Part print with two shaded views. Sizes in mm from the minimum x, y, z corner. A direction names the side the tool comes from. Give positions to 0.01 mm unless a question says otherwise; leave off trailing zeros. Order: outer loops, then holes, each group sorted by start corner. A loop starts at its lowest first (then second) coordinate and runs counter-clockwise, first axis right, second up. Notation, with made-up numbers: M -27,14 L 17,14 A13 ccw 17,20 Z; hole C 36.25,74.25 d8. An arc over 180 degrees is marked long. Answer as CSV lines item,"result".
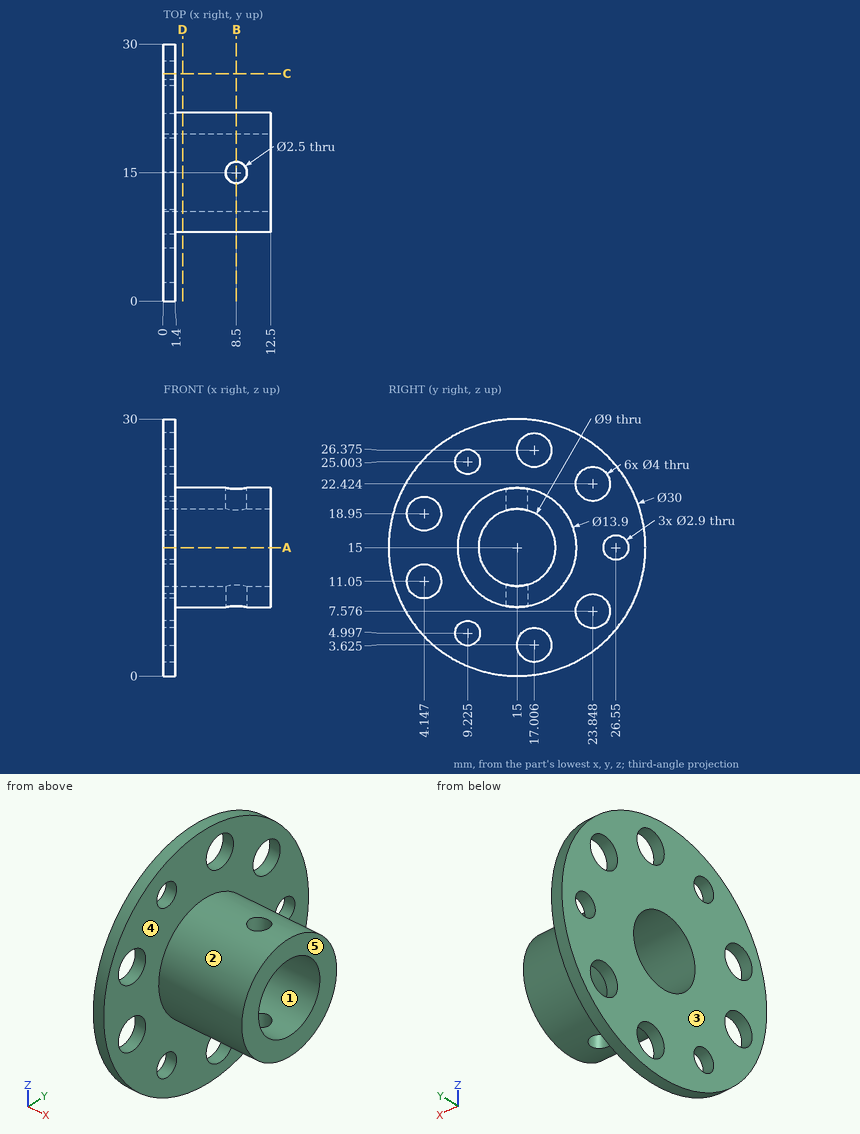
Item 1: 3-axis set-ups, long thin cutter, end or side, ignore diameter. For the marked faces 4 and 5: which of +Z, -Z, +X, -X, +Y, -Y reach the whole face in a straight line?
Geometry says:
face 4,"+X"
face 5,"+Z, -Z, +X, +Y, -Y"
Item 2: Probe line 1 along Y through (x, z) = (2.5, 15.25) (1 decimal); line 2 along X through (y, z) = (15, 9.7); line 3 along Z through (x, y) = (1.25, 13.25) (1 decimal). List the from-to ranges inside material, lowest first. Write a range as from..to.
Geometry says:
line 1,"y = 8.1..10.5, 19.5..21.9"
line 2,"x = 0..7.25, 9.75..12.5"
line 3,"z = 0.1..10.9, 19.1..29.9"
Item 3: Band-saw the part on A-A (z = 15). Give the cut face in (x, y).
Geometry says:
outline,"M 0,0 L 1.4,0 L 1.4,8.05 L 12.5,8.05 L 12.5,10.5 L 0,10.5 Z; M 0,19.5 L 12.5,19.5 L 12.5,21.95 L 1.4,21.95 L 1.4,25.1 L 0,25.1 Z; M 0,28 L 1.4,28 L 1.4,30 L 0,30 Z"
Item 4: Band-saw the part on C-C (y = 26.55). Give the cut face in (x, z).
Geometry says:
outline,"M 0,5.43 L 1.4,5.43 L 1.4,13.55 L 0,13.55 Z; M 0,16.45 L 1.4,16.45 L 1.4,24.57 L 0,24.57 Z"
Item 5: Drop flat-ended pins along their axis: pin 1 (6.5 mm diameter, centred on y = 4.15, z = 18.95, fed in from +X); pin 2 (3 mm diameter, centred on x = 8.5, y = 15, fed in from +Z); pin 3 (1 mm diameter, centred on x = 5, z = 21, fed in from -Y); pin 4 (11.5 mm diameter, centred on y = 15, z = 15, fed in from +X). Give the stop position or say it passes through.
Geometry says:
pin 1,"stops at x = 1.4"
pin 2,"stops at z = 21.95"
pin 3,"stops at y = 10.75"
pin 4,"stops at x = 12.5"
Item 6: Pull direction Z, two halves, no side cores. Call the marked faces 1, 2 and 3: released by +Z, released by -Z, zero draft, split by the parting line, or undercut.
Geometry says:
face 1,"undercut"
face 2,"split by the parting line"
face 3,"zero draft"
Item 7: Band-saw the part on D-D (x = 2.25). Give the cut face in (y, z).
Geometry says:
outline,"C 15,15 d13.9; hole C 15,15 d9"
Item 8: Band-saw the part on B-B (x = 8.5). Give the cut face in (y, z).
Geometry says:
outline,"M 13.75,8.16 L 13.75,10.68 A4.5 cw 13.75,19.32 L 13.75,21.84 A6.95 ccw Z; M 16.25,8.16 A6.95 ccw 16.25,21.84 L 16.25,19.32 A4.5 cw 16.25,10.68 Z"
